Design review of the part built by this model. Coordinates are the model's own, in mm. Face numbers are marked on the shaded views. A direction names the side the tool comes from. Give positions to 0.01 mm unless a question says otherwise; leave off trailing zeros. Loops run counter-clockwise (first coordinate to the right, second up) from the corner with the lowest first, then second, coordinate; pieces in that order, holes last. Notation, with made-up numbers: (53, 51.5) - (99, 51.5) arc R21 ccw to (99, 56.5) - close; hole circle Ø2 at (44, 80). An arc over 180 degrees is marked (long way). Write each question's results on one line, items separated by ' | '.
```python
from build123d import *

# Parameters (mm, degrees)
BOSS_EXTRUDE1_DEPTH = 15
BOSS_EXTRUDE2_DEPTH = 15
SKETCH3_W           = 20
SKETCH3_H           = 10
CUT_EXTRUDE1_DEPTH  = 15


with BuildPart() as part:
    # Sketch1 → Boss-Extrude1 (new body)
    with BuildSketch(Plane(origin=(0, 0, 0), x_dir=(1, 0, 0), z_dir=(0, 1, 0))):
        Polygon((0, 0), (30, 0), (30, 25), (70, 25), (70, 0), (100, 0), (100, 50), (0, 50), align=None)
    extrude(amount=BOSS_EXTRUDE1_DEPTH)

    # Sketch2 → Boss-Extrude2 (add)
    with BuildSketch(Plane(origin=(0, 15, 0), x_dir=(1, 0, 0), z_dir=(0, 1, 0))):
        Polygon((0, 0), (10, 0), (10, 40), (90, 40), (90, 0), (100, 0), (100, 50), (0, 50), align=None)
    extrude(amount=BOSS_EXTRUDE2_DEPTH)

    # Sketch3 → Cut-Extrude1 (cut)
    with BuildSketch(Plane(origin=(0, 30, 0), x_dir=(1, 0, 0), z_dir=(0, 1, 0))):
        with Locations((50, 45)):
            Rectangle(SKETCH3_W, SKETCH3_H)
    extrude(amount=-CUT_EXTRUDE1_DEPTH, mode=Mode.SUBTRACT)


solid = part.part
```
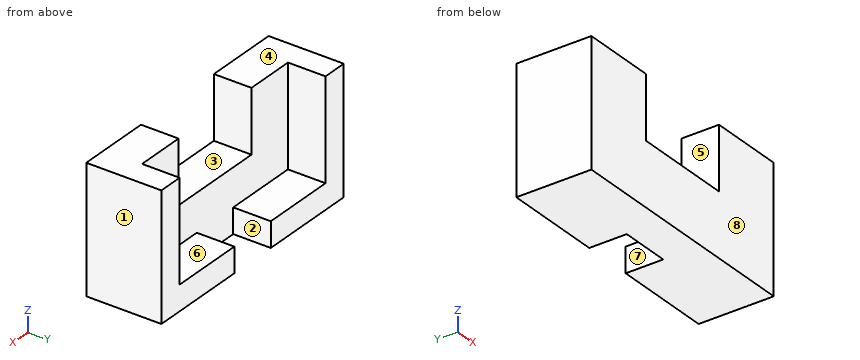
Item 1: We need section A-A on y = 19.25. Give the boundary of the cut face in (x, z), then the cut area to 3 significant figures.
Output values:
outline: (0, -50) - (40, -50) - (40, -40) - (10, -40) - (10, 0) - (0, 0) - close; (60, -50) - (100, -50) - (100, 0) - (90, 0) - (90, -40) - (60, -40) - close | area: 1,600 mm²
Item 2: We need section B-B on z = -19. Give the boundary of the cut face in (x, y).
Output values:
outline: (0, 0) - (30, 0) - (30, 15) - (10, 15) - (10, 30) - (0, 30) - close; (70, 0) - (100, 0) - (100, 30) - (90, 30) - (90, 15) - (70, 15) - close
Item 3: We need section C-C on z = -45. Give the boundary of the cut face in (x, y).
Output values:
outline: (0, 0) - (100, 0) - (100, 30) - (60, 30) - (60, 15) - (40, 15) - (40, 30) - (0, 30) - close
Item 4: We need section D-D on x = 82.5. Give the boundary of the cut face in (y, z).
Output values:
outline: (0, -50) - (30, -50) - (30, -40) - (15, -40) - (15, 0) - (0, 0) - close
Item 5: Draft analysis for pull direction X (two halves, no side actions). For the marked faces 1, 2, 3 and 4, state which applies: +X half, -X half, draft (parallel to the pull), parting line (faces both ways), or undercut.
Output values:
face 1: +X half | face 2: undercut | face 3: undercut | face 4: draft
Item 6: Clearance check with flat-ended pins moving along their axes: P1, Ø7.5, axis at x = 42.5, y = 8.5, coming from the +Z side; P2, Ø12, axis at x = 82, y = 24.5, coming from the +Z side; P3, Ø4, axis at x = 55.5, y = 18.5, coming from the -Z side. State where each tip first meets the part, or that it passes through.
Output values:
P1: stops at z = -25 | P2: stops at z = -40 | P3: passes through
Item 7: Wall thickness on probe 1 along X at (y, z) = (16, -1.5); probe 2 along X at (y, z) = (17.25, -44); probe 3 along Z at (x, y) = (61, 21.25): over which ranges is each line inside the solid? List them lowest first.
Output values:
probe 1: x = 0 to 10, 90 to 100 | probe 2: x = 0 to 40, 60 to 100 | probe 3: z = -50 to -40
Item 8: Tool access review of the marked faces 5, 6, 7 and 8: name each direction out of +Z, -Z, +X, -X, +Y, -Y from which nothing blocks a thin tool from reaching the whole face with its end or side.
Output values:
face 5: +Z, +Y, -Y | face 6: +Z, +Y | face 7: +Z, -Z, +Y | face 8: +Z, -Z, +X, -X, -Y
